The model under review builds one solid part; all positions refer to its coordinate system, in mm. Face numbers are marked on the shaded views. A direction names the side the tool comes from. Give positions to 0.01 mm unless a question says otherwise; leave off trailing zeros. Order: outer loops, then holes, each group sorted by start corner. A loop starts at its lowest first (then second) coordinate and runs counter-clockwise, first axis right, second up. Notation, with made-up numbers: (-37, 33) - (-14, 33) arc R29 cw to (-14, 69) - close; hole circle Ø7 at (87, 87). An arc over 180 degrees is marked (long way). Use a Markdown table: item, result. Add a question column.
```python
from build123d import *

# Parameters (mm, degrees)
EXTRUDE_1_DEPTH     = 12
SKETCH_2_W          = 5
SKETCH_2_H          = 2.5
CUT_EXTRUDE_1_DEPTH = 5
CUT_EXTRUDE_START   = -12
SKETCH_2_3_W        = 5
SKETCH_2_3_H        = 2.5
CUT_EXTRUDE_3_DEPTH = 5
SKETCH_2_4_R        = 2
CUT_EXTRUDE_4_DEPTH = 45.192307023
CUT_EXTRUDE_5_DEPTH = 11
SKETCH1_R           = 2.1
CUT_EXTRUDE1_DEPTH  = 43.560075188


with BuildPart() as part:
    # 草图1 → 凸台-拉伸1 (new body)
    with BuildSketch(Plane(origin=(0, 0, 0), x_dir=(1, 0, 0), z_dir=(0, 1, 0))):
        Polygon((0, 0), (0, 2), (15, 2), (15, 29.137304051), (12, 31.057304051), (0, 31.057304051), (0, 36.4), (12, 36.4), (22, 30), (22, 0), align=None)
    extrude(amount=EXTRUDE_1_DEPTH)

    # 草图2 → 切除-拉伸1 (cut)
    with BuildSketch(Plane.XZ):
        Polygon((12.5, -32.399476124), (12.5, -34.417827927), (19.9, -29.681827927), (19.9, -26), (16.4, -26), (16.4, -29.903476124), align=None)
        with Locations((18.5, -2.75)):
            Rectangle(SKETCH_2_W, SKETCH_2_H)
    extrude(amount=-CUT_EXTRUDE_1_DEPTH, mode=Mode.SUBTRACT)

    # 草图2<3> → 切除-拉伸3 (cut)
    with BuildSketch(Plane.XZ.offset(CUT_EXTRUDE_START)):
        Polygon((16.4, -26), (16.4, -29.903476124), (12.5, -32.399476124), (12.5, -34.417827927), (19.9, -29.681827927), (19.9, -26), align=None)
        with Locations((18.5, -2.75)):
            Rectangle(SKETCH_2_3_W, SKETCH_2_3_H)
    extrude(amount=CUT_EXTRUDE_3_DEPTH, mode=Mode.SUBTRACT)

    # 草图2<4> → 切除-拉伸4 (cut, through all)
    with BuildSketch(Plane.XZ):
        with Locations(Location((18.5, -23, 0), (0, 0, 270))):
            Circle(SKETCH_2_4_R)
        with Locations(Location((18.5, -7, 0), (0, 0, 270))):
            Circle(SKETCH_2_4_R)
    extrude(amount=-CUT_EXTRUDE_4_DEPTH, mode=Mode.SUBTRACT)

    # 草图2<5> → 切除-拉伸5 (cut)
    with BuildSketch(Plane.XZ):
        Polygon((1, -32.457304051), (1, -34.4), (11, -34.4), (11, -32.457304051), (9.25, -32.457304051), (9.25, -31.057304051), (2.75, -31.057304051), (2.75, -32.457304051), align=None)
        Polygon((17, -18.75), (17, -20), (20.2, -20), (20.2, -18.25), (22, -18.25), (22, -11.75), (20.2, -11.75), (20.2, -10), (17, -10), (17, -11.25), (17.5, -11.25), (17.5, -11.75), (17, -11.75), (17, -18.25), (17.5, -18.25), (17.5, -18.75), align=None)
    extrude(amount=-CUT_EXTRUDE_5_DEPTH, mode=Mode.SUBTRACT)

    # Sketch1 → Cut-Extrude1 (cut, through all)
    with BuildSketch(Plane(origin=(0, 0, -2), x_dir=(-1, 0, 0), z_dir=(0, 0, -1))):
        with Locations((-6, 6)):
            Circle(SKETCH1_R)
    extrude(amount=-CUT_EXTRUDE1_DEPTH, mode=Mode.SUBTRACT)


solid = part.part
```
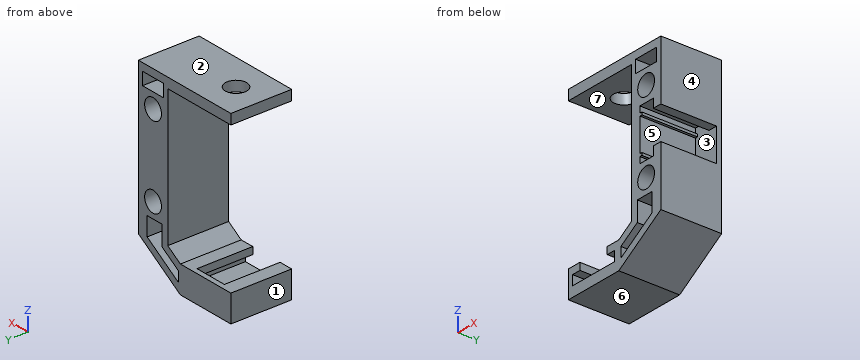
Q1. We need section B-B (z = -7). Write out the cut boundary in (x, y), plus the area to 3 significant figures.
Q2. We need section D-D (z = -27). Write out the cut boundary in (x, y), plus the area to 3 significant figures.
Q3. Clearance check with flat-ended pins moving along their axes: P1, Ø6, axis at x = 19.5, y = 3, coming from the -Z side; P2, Ø2.5, axis at x = 18, y = 3.5, coming from the -Z side; P3, Ø6, axis at y = 1.5, z = -19.5, coming from the -X side. State where each tip first meets the part, or that it passes through.
Q4. Draft analysis for pull direction X (two halves, no side actions). For the marked faces 1, 2, 3 and 4, state which applies: pulls with the +X half, pulls with the -X half, needs draft (parallel to the pull), parting line crosses it, or undercut.
Q5. We need section C-C (x = 10.5). Write out the cut boundary in (y, z).
Q6. We need section A-A (x = 6). Write out the cut boundary in (y, z).
Q7. Wall thickness on probe 1 along Z at (x, y) = (9.5, 1); probe 2 along Z at (x, y) = (3.25, 10.25); probe 3 along X at (y, z) = (11.25, -27.5): over which ranges is each line inside the solid? List them lowest first.
Q8. Machinability: for the marked faces 5, 6 and 7, which of the approach directions +Z, -Z, +X, -X, +Y, -Y give a long, thin tool a straight path to every point of the face, cutting with its end or side? Answer none if there is none.
Here are the results:
| question | item | result |
|---|---|---|
| 1 | outline | (15, 0) - (16.5, 0) - (16.5, 12) - (15, 12) - close; (20.5, 0) - (22, 0) - (22, 12) - (20.5, 12) - close |
| 1 | area | 36.0 mm2 |
| 2 | outline | (15, 0) - (16.4, 0) - (16.4, 5) - (19.9, 5) - (19.9, 0) - (22, 0) - (22, 12) - (19.9, 12) - (19.9, 7) - (16.4, 7) - (16.4, 12) - (15, 12) - close |
| 2 | area | 49.0 mm2 |
| 3 | P1 | z = -33.52 |
| 3 | P2 | z = -33.36 |
| 3 | P3 | x = 15 |
| 4 | face 1 | pulls with the -X half |
| 4 | face 2 | needs draft |
| 4 | face 3 | undercut |
| 4 | face 4 | pulls with the +X half |
| 5 | outline | (0, -36.4) - (12, -36.4) - (12, -31.06) - (0, -31.06) - (0, -32.46) - (11, -32.46) - (11, -34.4) - (0, -34.4) - close; (0, -2) - (12, -2) - (12, 0) - (0, 0) - close |
| 6 | outline | (0, -36.4) - (12, -36.4) - (12, -31.06) - (11, -31.06) - (11, -34.4) - (0, -34.4) - close; (0, -2) - (3.9, -2) - (3.9, 0) - (0, 0) - close; (8.1, -2) - (12, -2) - (12, 0) - (8.1, 0) - close |
| 7 | probe 1 | -36.4 to -34.4, -32.46 to -31.06, -2 to 0 |
| 7 | probe 2 | -36.4 to -34.4, -2 to 0 |
| 7 | probe 3 | 15 to 16.4, 19.9 to 22 |
| 8 | face 5 | +X, -Y |
| 8 | face 6 | -Z, +X, -X, +Y, -Y |
| 8 | face 7 | -X, +Y, -Y |
